Autodesk Inventor part; units mm, degrees
ref_plane "YZ Plane" through (0, 0, 0) normal (1, 0, 0) x (0, 1, 0)
ref_plane "XZ Plane" through (0, 0, 0) normal (0, 1, 0) x (-1, 0, 0)
ref_plane "XY Plane" through (0, 0, 0) normal (0, 0, 1) x (1, 0, 0)
sketch "Sketch1" plane through (0, 0, 0) normal (0, 1, 0) x (-1, 0, 0)
  line L0 (0, 0) -> (0, -44)
  line L1 (0, -44) -> (85, -44)
  line L2 (85, -44) -> (85, 0)
  line L3 (85, 0) -> (0, 0)
  line L4 (0, -46) -> (-2, -46)
  line L5 (-2, -46) -> (-2, 0)
  line L6 (-2, 0) -> (-2, 2)
  line L7 (-2, 2) -> (85, 2)
  line L8 (85, 2) -> (87, 2)
  line L9 (87, 2) -> (87, -46)
  line L10 (87, -46) -> (0, -46)
  dimension "d0" = 44
  dimension "d2" = 2
  dimension "d3" = 2
  dimension "d4" = 2
  dimension "d5" = 2
extrude "Extrusion1" add sketch "Sketch1" along normal blind 2 contours L3 L2 L1 L0 | L4 L5 L6 L7 L8 L9 L10
extrude "Extrusion2" add sketch "Sketch1" against normal blind 25
sketch "Sketch2" plane through (2, 2, 2) normal (1, 0, 0) x (0, 0, -1)
  point P0 (2, -2)
sketch "Sketch3" plane through (2, 2, 2) normal (1, 0, 0) x (0, 0, -1)
  line L0 (0, -27) -> (13.1, -27)
  line L1 (46, -27) -> (2, -27)
  line L2 (0, -27) -> (48, -27)
  line L3 (48, -27) -> (34.9, -27)
  line L4 (34.9, -27) -> (34.9, -7)
  line L5 (34.9, -7) -> (13.1, -7)
  line L6 (13.1, -7) -> (13.1, -27)
  line L7 (13.1, -27) -> (34.9, -27)
  point P0 (2, -2)
  dimension "d10" = 13.1
  dimension "d11" = 13.1
  dimension "d12" = 20
extrude "Extrusion3" cut sketch "Sketch3" against normal blind 25
fillet "Fillet1" radius 2 5 edges at (-42.5, 2, -46) (2, -11.5, -46) (2, 2, -22) (-87, 2, -22) (-87, -11.5, -46)
sketch "Sketch4" plane through (-87, -25, 2) normal (0, 0, 1) x (1, 0, 0)
  line L0 (2, 0) -> (0, 0)
  line L1 (0, 0) -> (7.4, 0)
  line L2 (87, 0) -> (2, 0)
  line L3 (7.4, 0) -> (15.2, 0)
  line L4 (15.2, 0) -> (15.2, 6)
  line L5 (15.2, 6) -> (7.4, 6)
  line L6 (7.4, 6) -> (7.4, 0)
  point P0 (87, 25)
  dimension "d16" = 7.4
  dimension "d17" = 7.8
  dimension "d18" = 6
extrude "Extrusion4" cut sketch "Sketch4" against normal blind 25
sketch "Sketch5" plane through (0, 2, 0) normal (0, 1, 0) x (1, 0, 0)
  line L0 (2, 32.9) -> (0, 32.9)
  line L1 (0, 11.1) -> (2, 11.1)
  line L2 (0, 32.9) -> (0, 11.1)
  line L3 (0, 11.1) -> (-2, 11.1)
  line L4 (-2, 11.1) -> (-6, 11.1)
  line L5 (-6, 11.1) -> (-6, 32.9)
  line L6 (-6, 32.9) -> (-2, 32.9)
  line L7 (-2, 32.9) -> (-2, 11.1)
  point P0 (0, 0)
  dimension "d21" = 2
  dimension "d22" = 4
  dimension "d23" = 4
extrude "Extrusion5" cut sketch "Sketch5" against normal blind 0.5
sketch "Sketch6" plane through (-87, -25, -44) normal (-1, 0, 0) x (0, 0, 1)
  line L0 (46, 25) -> (0, 25)
  line L1 (23, 25) -> (23, 0)
  line L2 (46, 0) -> (0, 0)
  line L3 (23, 0) -> (28, 0)
  line L4 (28, 0) -> (28, 5)
  line L5 (28, 5) -> (18, 5)
  line L6 (18, 5) -> (18, 0)
  line L7 (23, 0) -> (18, 0)
  point P0 (44, 25)
  dimension "d26" = 5
  dimension "d27" = 5
  dimension "d28" = 10
extrude "Extrusion6" add sketch "Sketch6" along normal blind 2
sketch "Sketch7" plane through (0, -25, 0) normal (0, -1, 0) x (1, 0, 0)
  line L0 (-87, -44) -> (-87, 2)
  line L1 (-87, -26) -> (-89, -26)
  line L2 (-87, -15.9645) -> (-87, -26)
  line L3 (-87, -26) -> (-89, -26)
  line L4 (-89, -26) -> (-89, -16)
  line L5 (-89, -26) -> (-89, -16)
  line L6 (-87, -16) -> (-89, -16)
  line L7 (-89, -16) -> (-87, -16)
  point P0 (0, 0)
extrude "Extrusion7" add sketch "Sketch7" along normal blind 10
sketch "Sketch8" plane through (-89, -25, -44) normal (-1, 0, 0) x (0, 0, 1)
  line L0 (28, 0) -> (18, 0)
  line L1 (18, 0) -> (23, 0)
  line L2 (23, 0) -> (23, -5)
  circle A0 centre (23, -5) radius 1.6
  point P0 (44, 25)
  dimension "d33" = 5
  dimension "d34" = 3.2
extrude "Extrusion8" cut sketch "Sketch8" against normal blind 10
sketch "Sketch9" plane through (2, -25, -11.1) normal (1, 0, 0) x (0, 0, -1)
  line L0 (-13.1, 0) -> (4.9, 0)
  line L1 (-13.1, 0) -> (-11.1, 0)
  line L2 (-11.1, 0) -> (-11.1, 5)
  line L3 (-11.1, 6) -> (-11.1, 0)
  line L4 (-11.1, 5) -> (-1.1, 5)
  line L5 (-1.1, 5) -> (-1.1, 0)
  line L6 (-1.1, 0) -> (-11.1, 0)
  line L7 (32.9, 0) -> (-11.1, 0)
  line L8 (32.9, 0) -> (32.9, 5)
  line L9 (32.9, 0) -> (32.9, 25)
  line L10 (32.9, 5) -> (22.9, 5)
  line L11 (22.9, 5) -> (22.9, 0)
  line L12 (22.9, 0) -> (32.9, 0)
  point P0 (-11.1, 25)
  dimension "d37" = 2
  dimension "d38" = 5
  dimension "d39" = 10
  dimension "d40" = 5
  dimension "d41" = 10
extrude "Extrusion9" add sketch "Sketch9" along normal blind 2
sketch "Sketch10" plane through (0, -25, 0) normal (0, -1, 0) x (1, 0, 0)
  line L0 (4, -10) -> (4, 0)
  line L1 (2, -10) -> (4, -10)
  line L2 (4, -10) -> (2, -10)
  line L3 (2, 0) -> (2, -10)
  line L4 (2, -10) -> (2, 0)
  line L5 (2, 0) -> (4, 0)
  line L6 (4, 0) -> (4, -10)
  line L7 (4, -44) -> (4, -34)
  line L8 (4, -34) -> (4, -44)
  line L9 (2, -44) -> (4, -44)
  line L10 (4, -44) -> (2, -44)
  line L11 (2, -44) -> (2, -34)
  line L12 (2, 2) -> (2, -44)
  line L13 (4, -34) -> (2, -34)
  point P0 (0, 0)
extrude "Extrusion10" add sketch "Sketch10" along normal blind 10
sketch "Sketch11" plane through (4, -25, -11.1) normal (1, 0, 0) x (0, 0, -1)
  line L0 (-1.1, -10) -> (-11.1, -10)
  line L1 (-6.1, -10) -> (-6.1, -5)
  line L2 (22.9, -10) -> (32.9, -10)
  line L3 (27.9, -10) -> (27.9, -5)
  circle A0 centre (-6.1, -5) radius 1.6
  circle A1 centre (27.9, -5) radius 1.6
  point P0 (-11.1, 25)
  dimension "d46" = 5
  dimension "d47" = 5
  dimension "d48" = 3.2
  dimension "d49" = 3.2
extrude "Extrusion11" cut sketch "Sketch11" against normal blind 10
sketch "Sketch12" plane through (0, 0, 0) normal (0, 0, -1) x (-1, 0, 0)
  line L0 (0, -5) -> (0, -25)
  line L1 (71.8, -19) -> (71.8, -25)
  line L2 (0, -25) -> (71.8, -25)
  line L3 (71.8, -25) -> (71.8, -23)
  line L4 (71.8, -23) -> (0, -23)
  line L5 (0, -23) -> (0, -25)
  point P0 (0, 0)
  dimension "d52" = 2
extrude "Extrusion12" add sketch "Sketch12" along normal blind 2
sketch "Sketch13" plane through (-85, 0, -44) normal (0, 0, 1) x (1, 0, 0)
  line L0 (87, -25) -> (13.2, -25)
  line L1 (13.2, -23) -> (85, -23)
  line L2 (13.2, -25) -> (13.2, -23)
  line L3 (13.2, -23) -> (85, -23)
  line L4 (85, -5) -> (85, -25)
  line L5 (85, -23) -> (85, -25)
  line L6 (85, -25) -> (13.2, -25)
  point P0 (85, 0)
extrude "Extrusion13" add sketch "Sketch13" along normal blind 2
properties part number "sideboard_top"
Model file for the job. Use its own axes, mm. A direction names the side the tool comes from. Give positions to 0.01 mm unless a question says otherwise; leave off trailing zeros. Loops run counter-clockwise (first coordinate to the right, second up) from the corner with the lowest first, then second, coordinate; pieces in that order, holes last. Notation, with made-up numbers: (-35.5, 24.25) - (-18.5, 24.25) arc R25 cw to (-18.5, 44.25) - close; hole circle Ø11 at (51, -22.5). An arc over 180 degrees is marked (long way). One line per item, written item: value. Start each with the question number.
1. Which spindle directions (+Z, -Z, +X, -X, +Y, -Y) get a long thin tool onto all of the face, cutting with end or side? Do faces 1 (the flat face through (-88, -27, -16)), 2 (the flat face through (-4, 1.5, -22)), 3 (the flat face through (3, -27, -34)). Say none if no direction does.
2. Slice it at A-A (y = -30). List the corners of the cut face in (x, z).
3. Slice it at D-D (z = -36.5). List the corners of the cut face in (x, y).
4. Slice it at C-C (x = -8). List the corners of the cut face in (y, z).
5. Slice it at B-B (z = -21). List the corners of the cut face in (x, y).
6. Pull direction X, two halves, no side cores. Call faces 4 (the flat face through (4, -27, -5)), 5 (the flat face through (3, -27, -10)), 6 (the flat face through (-36, -24, -42)), 7 (the flat face through (-35, -24, -2)): pulls with the +X half, pulls with the -X half, needs draft (parallel to the pull), parting line crosses it, or undercut.
7. Pin check, flat tips, straight feed: pin 1 (1.2 mm diameter, centred on y = -23, z = -1, fed in from -X); pin 2 (0.6 mm diameter, centred on x = 2.5, y = -27, fed in from +Z); pin 3 (6.5 mm diameter, centred on x = -27, z = -7.5, fed in from -Y). Stop position of each tip, or through.
8. Probe L1, parallel to Z at x = 3, y = -30; L2, parallel to X at y = -16, z = -7; L3, parallel to Z at x = -54.5, y = -24. List the from-to ranges inside material, lowest first. Write a range as from..to.
Solution:
1. face 1: +Z, -X, +Y, -Y
1. face 2: +Y
1. face 3: +X, +Y, -Y
2. outline: (-89, -26) - (-87, -26) - (-87, -22.6) - (-89, -22.6) - close; (-89, -19.4) - (-87, -19.4) - (-87, -16) - (-89, -16) - close; (2, -44) - (4, -44) - (4, -40.6) - (2, -40.6) - close; (2, -37.4) - (4, -37.4) - (4, -34) - (2, -34) - close; (2, -10) - (4, -10) - (4, -6.6) - (2, -6.6) - close; (2, -3.4) - (4, -3.4) - (4, 0) - (2, 0) - close
3. outline: (-87, -25) - (-85, -25) - (-85, 0) - (0, 0) - (0, -25) - (2, -25) - (2, -35) - (4, -35) - (4, -20) - (2, -20) - (2, 0) arc R2 ccw to (0, 2) - (-85, 2) arc R2 ccw to (-87, 0) - close
4. outline: (-25, -46) - (0, -46) arc R2 ccw to (2, -44) - (2, 2) - (-25, 2) - (-25, -2) - (-23, -2) - (-23, 0) - (0, 0) - (0, -44) - (-23, -44) - (-23, -42) - (-25, -42) - close
5. outline: (-89, -35) - (-87, -35) - (-87, -31.6) - (-89, -31.6) - close; (-89, -28.4) - (-87, -28.4) - (-87, -25) - (-85, -25) - (-85, 0) - (0, 0) - (0, -5) - (2, -5) - (2, 0) arc R2 ccw to (0, 2) - (-2, 2) - (-2, 1.5) - (-6, 1.5) - (-6, 2) - (-85, 2) arc R2 ccw to (-87, 0) - (-87, -20) - (-89, -20) - close
6. face 4: pulls with the +X half
6. face 5: needs draft
6. face 6: undercut
6. face 7: undercut
7. pin 1: stops at x = -87
7. pin 2: stops at z = 0
7. pin 3: stops at y = 0
8. L1: z = -44..-40.6, -37.4..-34, -10..-6.6, -3.4..0
8. L2: x = -87..-85, 0..2
8. L3: z = -46..-42, -2..2
